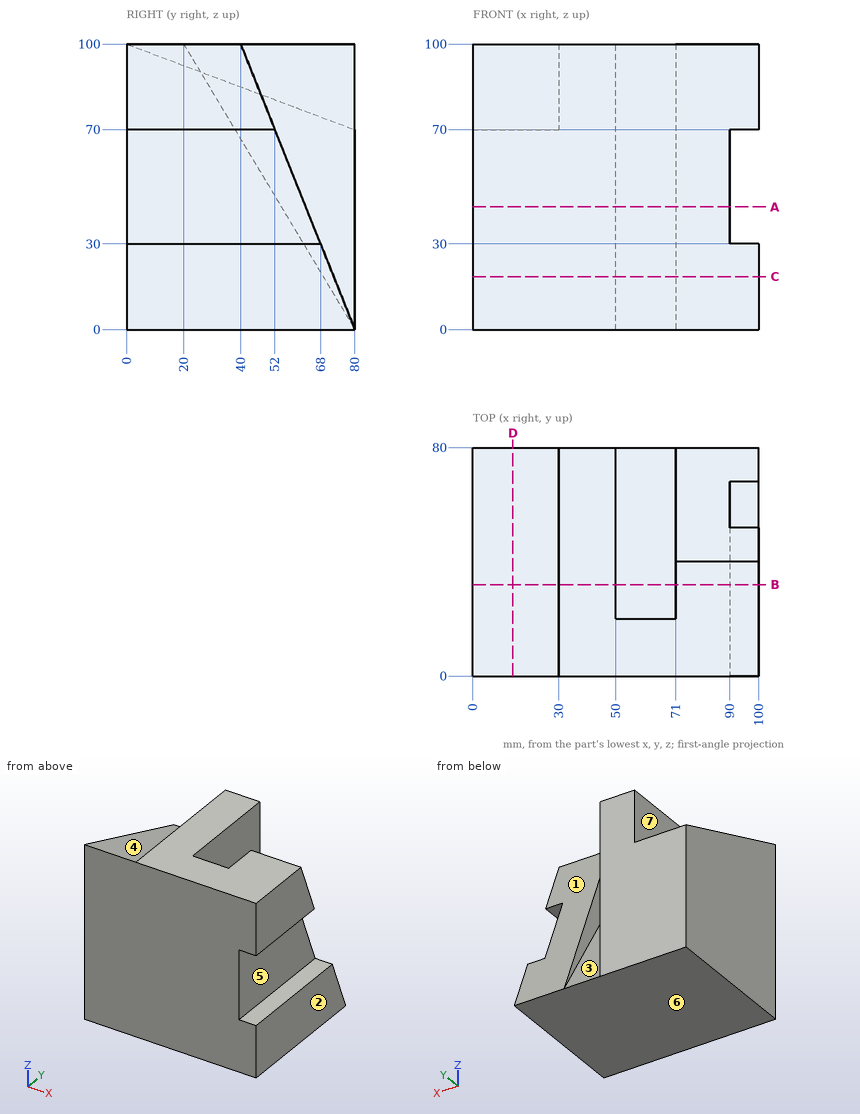
For this review, use the dimensioned drawing (mm, ordinates from the lowest corner) and the shaded views. A direction names the side the tool comes from. Give positions to 0.01 mm unless a question says otherwise; leave off trailing zeros. Order: outer loops, then holes, each group sorted by start corner. A loop starts at its lowest first (then second) coordinate and runs counter-clockwise, first axis right, second up.
1. Add section B-B, the plane y = 32. State the section outline as (x, z) points, then the cut area to 3 significant figures.
Solution:
outline: (0, 0) - (100, 0) - (100, 30) - (90, 30) - (90, 70) - (100, 70) - (100, 100) - (71, 100) - (71, 80) - (50, 80) - (50, 100) - (30, 100) - (30, 88) - (0, 88) - close
area: 8,820 mm2
2. Add section D-D, the plane x = 14. State the section outline as (y, z) points.
Solution:
outline: (0, 0) - (80, 0) - (80, 70) - (0, 100) - close
3. Tool access review of the marked faces 1, 2, 3 and 4: name each direction out of +Z, -Z, +X, -X, +Y, -Y from which nothing blocks a thin tool from reaching the whole face with its end or side.
Solution:
face 1: +Z, +X, +Y
face 2: +Z, -Z, +X, +Y, -Y
face 3: +Z, +Y
face 4: +Z, -X, +Y
4. Add section A-A, the plane z = 43. State the section outline as (x, y) points, then the cut area to 3 significant figures.
Solution:
outline: (0, 0) - (90, 0) - (90, 62.8) - (71, 62.8) - (71, 54.2) - (50, 54.2) - (50, 80) - (0, 80) - close
area: 6,330 mm2
5. Add section C-C, the plane z = 18.5. State the section outline as (x, y) points.
Solution:
outline: (0, 0) - (100, 0) - (100, 72.6) - (71, 72.6) - (71, 68.9) - (50, 68.9) - (50, 80) - (0, 80) - close
6. For pin 1 Ø5 at (y, z) = (35, 49) entering from +X; pin 2 Ø10 at (x, z) = (62.5, 51.5) entering from +Y; pin 3 Ø6 at (x, y) = (12, 45.5) entering from +Z, all flat-tipped, find the tip position at first contact; note any pin that passes through.
Solution:
pin 1: stops at x = 90
pin 2: stops at y = 52.1
pin 3: stops at z = 84.06
7. Mouldability with a two-part tool opening along Z and no side actions: class the marked faces 5, 6 and 7 as +Z half, -Z half, draft (parallel to the pull), parting line (faces both ways), or undercut.
Solution:
face 5: undercut
face 6: -Z half
face 7: draft
8. To check wall thickness, follow L1, parallel to X at y = 32.5, z = 88; L2, parallel to Z at x = 90.5, y = 17; L3, parallel to X at y = 55, z = 85.5. State the ranges of each line that lie inside material, in increasing order.
Solution:
L1: x = 30 to 50, 71 to 100
L2: z = 0 to 30, 70 to 100
L3: x = 30 to 50
